Verification items for the finished model (mm, model axes). A direction names the side the tool comes from. Round coordinates to 2 decimals unless told otherwise and drop trailing zeros. Order: outer loops, then holes, each group sorted by start corner. A loop starts at its lowest first (then second) coordinate and runs counter-clockwise, first axis right, second up. Notation, with made-up numbers: M -32.5,-14.5 L -21.5,-14.5 A13 ccw -21.5,7.5 Z; hole C -31,-13 d10. An arc over 180 degrees is marked long. One line per item, written item: value. Start each with the question number.
from build123d import *

# Parameters (mm, degrees)
ESBO_O1_R                = 1.75
RESSALTO_EXTRUS_O1_DEPTH = 4
ESBO_O2_W                = 35
ESBO_O2_H                = 20
CORTE_EXTRUS_O1_DEPTH    = 111.962426073
ESBO_O3_W                = 217
ESBO_O3_H                = 1.79
RESSALTO_EXTRUS_O2_DEPTH = 4
ESBO_O4_W                = 27
ESBO_O4_H                = 6
CORTE_EXTRUS_O2_DEPTH    = 111.962426073
ESBO_O5_W                = 163
ESBO_O5_H                = 1
CORTE_EXTRUS_O3_DEPTH    = 111.962426073
ESBO_O6_R                = 2.1
RESSALTO_EXTRUS_O4_DEPTH = 4
FILETE1_R                = 5
FILETE2_R                = 5


with BuildPart() as part:
    # Esboço1 → Ressalto-extrusão1 (new body)
    with BuildSketch(Plane(origin=(0, 0, 0), x_dir=(0, 0, -1), z_dir=(1, 0, 0))):
        Polygon((-108.5, 18.9), (108.5, 18.9), (108.5, 10), (103.5, 10), (103.5, 5), (108.5, 5), (108.5, -5), (103.5, -5), (103.5, -10), (108.5, -10), (108.5, -18.9), (73.5, -18.9), (73.5, -22.9), (68.5, -22.9), (68.5, -18.9), (65.25, -18.9), (65.25, -12.65), (67.75, -12.65), (67.75, -7.15), (65.25, -7.15), (65.25, -2.9), (61.75, -2.9), (61.75, -7.15), (59.25, -7.15), (59.25, -12.65), (61.75, -12.65), (61.75, -18.9), (58.5, -18.9), (58.5, -22.9), (53.5, -22.9), (53.5, -18.9), (-53.5, -18.9), (-53.5, -22.9), (-58.5, -22.9), (-58.5, -18.9), (-61.75, -18.9), (-61.75, -12.65), (-59.25, -12.65), (-59.25, -7.15), (-61.75, -7.15), (-61.75, -2.9), (-65.25, -2.9), (-65.25, -7.15), (-67.75, -7.15), (-67.75, -12.65), (-65.25, -12.65), (-65.25, -18.9), (-68.5, -18.9), (-68.5, -22.9), (-73.5, -22.9), (-73.5, -18.9), (-108.5, -18.9), (-108.5, -10), (-103.5, -10), (-103.5, -5), (-108.5, -5), (-108.5, 5), (-103.5, 5), (-103.5, 10), (-108.5, 10), align=None)
        with Locations((-105.5, 0)):
            Circle(ESBO_O1_R, mode=Mode.SUBTRACT)
        with Locations(Location((105.5, 0, 0), (0, 0, 180))):
            Circle(ESBO_O1_R, mode=Mode.SUBTRACT)
    extrude(amount=RESSALTO_EXTRUS_O1_DEPTH)

    # Esboço2 → Corte-extrusão1 (cut, through all)
    with BuildSketch(Plane(origin=(4, 0, 0), x_dir=(0, 0, -1), z_dir=(1, 0, 0))):
        Rectangle(ESBO_O2_W, ESBO_O2_H)
    extrude(amount=-CORTE_EXTRUS_O1_DEPTH, mode=Mode.SUBTRACT)

    # Esboço3 → Ressalto-extrusão2 (add, through all)
    with BuildSketch(Plane(origin=(4, 0, 0), x_dir=(0, 0, -1), z_dir=(1, 0, 0))):
        with Locations((0, 19.795)):
            Rectangle(ESBO_O3_W, ESBO_O3_H)
    extrude(amount=-RESSALTO_EXTRUS_O2_DEPTH)

    # Esboço4 → Corte-extrusão2 (cut, through all)
    with BuildSketch(Plane(origin=(4, 0, 0), x_dir=(0, 0, -1), z_dir=(1, 0, 0))):
        with Locations((-95, 17.69)):
            Rectangle(ESBO_O4_W, ESBO_O4_H)
        with Locations((95, 17.69)):
            Rectangle(ESBO_O4_W, ESBO_O4_H)
    extrude(amount=-CORTE_EXTRUS_O2_DEPTH, mode=Mode.SUBTRACT)

    # Esboço5 → Corte-extrusão3 (cut, through all)
    with BuildSketch(Plane(origin=(4, 0, 0), x_dir=(0, 0, -1), z_dir=(1, 0, 0))):
        with Locations((0, 20.19)):
            Rectangle(ESBO_O5_W, ESBO_O5_H)
    extrude(amount=-CORTE_EXTRUS_O3_DEPTH, mode=Mode.SUBTRACT)

    # Esboço6 → Ressalto-extrusão4 (add, through all)
    # profile 1 of 2: a face of its own
    with BuildSketch(Plane(origin=(4, 0, 0), x_dir=(0, 0, -1), z_dir=(1, 0, 0))):
        with BuildLine():
            Line((-57, 19.69), (-57, 30.82))
            ThreePointArc((-57, 30.82), (-55.535533906, 34.355533906), (-52, 35.82))
            Line((-52, 35.82), (-48, 35.82))
            ThreePointArc((-48, 35.82), (-44.464466094, 34.355533906), (-43, 30.82))
            Line((-43, 30.82), (-43, 19.69))
            Line((-43, 19.69), (-57, 19.69))
        make_face()
        with Locations((-50, 29.82)):
            Circle(ESBO_O6_R, mode=Mode.SUBTRACT)
    # profile 2 of 2: a face of its own
    with BuildSketch(Plane(origin=(4, 0, 0), x_dir=(0, 0, -1), z_dir=(1, 0, 0))):
        with BuildLine():
            Line((43, 30.82), (43, 19.69))
            Line((43, 19.69), (57, 19.69))
            Line((57, 19.69), (57, 30.82))
            ThreePointArc((57, 30.82), (55.535533906, 34.355533906), (52, 35.82))
            Line((52, 35.82), (48, 35.82))
            ThreePointArc((48, 35.82), (44.464466094, 34.355533906), (43, 30.82))
        make_face()
        with Locations(Location((50, 29.82, 0), (0, 0, 180))):
            Circle(ESBO_O6_R, mode=Mode.SUBTRACT)
    extrude(amount=-RESSALTO_EXTRUS_O4_DEPTH)

    # Filete1
    filete1_edges = [part.edges().sort_by_distance(p)[0] for p in [
        (2, 19.69, 43),
        (2, 19.69, 57),
        (2, 19.69, -57),
        (2, 19.69, -43),
    ]]
    fillet(filete1_edges, radius=FILETE1_R)

    # Filete2
    filete2_edges = [part.edges().sort_by_distance(p)[0] for p in [
        (2, 10, -17.5),
        (2, -10, -17.5),
        (2, -10, 17.5),
        (2, 10, 17.5),
    ]]
    fillet(filete2_edges, radius=FILETE2_R)


solid = part.part
1. Draft check along Z on faces 5 (the face through (1.97, 21.12, -41.5)), 6 (the face through (2, -5, -106)), 7 (the face through (2, -15, 108.5)). Enter one of: released by +Z, released by -Z, zero draft, split by the parting line, or undercut.
2. Section check A-A (z = -0.5). Record the cut outline in (x, y).
3. Section check C-C (x = 2.8). Give the number of separate pieces and of enclosed holes in the cut face, and give its area (3 significant figures).
4. Depth check by flat-ended pin: pin 1 (1.2 mm diameter, centred on x = 2.5, y = 27.5, fed in from -Z); pin 2 (1.2 mm diameter, centred on x = 2.5, z = -68, fed in from +Y); pin 3 (1 mm diameter, centred on x = 1.5, y = 9, fed in from -Z). Enter the tip coordinate at first touch or a pass-through.
5. Section check B-B (y = 8). Record the cut outline in (x, z), and give its area (3 significant figures).
6. Tool access check on faces 1 (the face through (2, 28, 43)), 2 (the face through (2, 7, 103.5)), 3 (the face through (1.97, 8.57, -16)), 4 (the face through (2, -2.9, 63)). Record the directions out of +Z, -Z, +X, -X, +Y, -Y that give a thin tool (end or side, any length) a straight path to the whole face; none if there is none.
7. Scan lines: line 1 along Z through (x, y) = (3.4, -18); line 2 along Y through (x, z) = (3, -105.5); line 3 along Z through (x, y) = (2.15, 30). Record each from-to range of solid material in increasing order.
8. Section check D-D (z = -30). Record the cut outline in (x, y).
Geometry check:
1. face 5: undercut
1. face 6: zero draft
1. face 7: released by +Z
2. outline: M 0,-18.9 L 4,-18.9 L 4,-10 L 0,-10 Z; M 0,10 L 4,10 L 4,19.69 L 0,19.69 Z
3. separate pieces: 1
3. enclosed holes: 5
3. area: 7,640 mm²
4. pin 1: stops at z = -57
4. pin 2: stops at y = 19.69
4. pin 3: stops at z = -103.5
5. outline: M 0,-103.5 L 4,-103.5 L 4,-16.5 L 0,-16.5 Z; M 0,16.5 L 4,16.5 L 4,103.5 L 0,103.5 Z
5. area: 696 mm²
6. face 1: +X, -X, +Y
6. face 2: +Z, +X, -X
6. face 3: +X, -X
6. face 4: +X, -X, -Y
7. line 1: z = -108.5 to -65.25, -61.75 to 61.75, 65.25 to 108.5
7. line 2: y = -18.9 to -10, -5 to -1.75, 1.75 to 5, 10 to 14.69
7. line 3: z = -57 to -52.09, -47.91 to -43, 43 to 47.91, 52.09 to 57
8. outline: M 0,-18.9 L 4,-18.9 L 4,19.69 L 0,19.69 Z
